```python
from build123d import *

# Parameters (mm, degrees)
F1_DEPTH = 30
F2_T     = -1
F3_DEPTH = 1


with BuildPart() as f1:
    # F0 (on Top) → F1 (new body)
    with BuildSketch(Plane.XY):
        Polygon((0, -120), (0, 0), (-25, 0), (-25, -35), (-25, -60), (-25, -100), (-25, -120), align=None)
        Polygon((0, -180), (0, -120), (-25, -120), (-25, -125), (-25, -180), align=None)
        Polygon((-25, -60), (-25, -35), (-145, -35), (-145, -60), (-110, -60), (-85, -60), align=None)
        Polygon((-25, -125), (-25, -120), (-25, -100), (-85, -100), (-85, -120), (-85, -125), align=None)
        Polygon((-85, -100), (-85, -60), (-110, -60), (-110, -120), (-85, -120), align=None)
    extrude(amount=F1_DEPTH)

    # F2
    f2_openings = [f1.faces().sort_by_distance(p)[0] for p in [
        (-12.5, -180, 15),
    ]]
    offset(amount=F2_T, openings=f2_openings, kind=Kind.INTERSECTION)

    # F3 (cut): a face of the model
    f3_faces = [f1.faces().sort_by_distance(p)[0] for p in [
        (-12.5, -2.3113848663, 30),
    ]]
    extrude(f3_faces, amount=-F3_DEPTH, mode=Mode.SUBTRACT)


solid = f1.part
```
Could you check a few things on this model? Use its own coordinates, in mm. A direction names the side the tool comes from. Round coordinates to 2 decimals unless told otherwise and drop trailing zeros. Loops run counter-clockwise (first coordinate to the right, second up) from the corner with the lowest first, then second, coordinate; pieces in that order, holes last. Notation, with made-up numbers: M 67,-3.5 L 121,-3.5 A8 ccw 121,11.5 Z; hole C -4.75,-11.75 d10. An arc over 180 degrees is marked long. Put each result on its own line as item: value.
Q1. Imagine slicing it at D-D (y = -68.5). Write out the boundary of the cut face in (x, z), then the cut area to 3 significant figures.
Check result:
outline: M -110,0 L -85,0 L -85,29 L -86,29 L -86,1 L -109,1 L -109,29 L -110,29 Z; M -25,0 L 0,0 L 0,29 L -1,29 L -1,1 L -24,1 L -24,29 L -25,29 Z
area: 162 mm2
Q2. On a 3-axis mill with a long thin cutter (end or side, diameter ignored), from which of +Z, -Z, +X, -X, +Y, -Y can I reach the whole of each face in a straight line? I mean faces 1 (the face through (-128, -60, 14)), 2 (the face through (-83, -36, 15)), 3 (the face through (-84, -35, 14)), 4 (the face through (-25, -80, 14)). Say none if no direction works.
Check result:
face 1: +Z, -Z, -X, -Y
face 2: +Z
face 3: +Z, -Z, -X, +Y
face 4: +Z, -Z
Q3. Imagine slicing it at A-A (z = 4.5). State how many separate pieces and enclosed holes the cut face has, then the cut area to 3 significant figures.
Check result:
separate pieces: 2
enclosed holes: 1
area: 827 mm2
Q4. For pin 1 (5 mm diameter, centred on y = -155.5, z = 9.5, fed in from -X); pin 2 (7.5 mm diameter, centred on x = -95.5, z = 7.5, fed in from -Y); pin 3 (14.5 mm diameter, centred on y = -74.5, z = 12, fed in from -X), each with a flat end and sliding along its axis, tell me the tip position at first contact or that it passes through.
Check result:
pin 1: x = -25
pin 2: y = -120
pin 3: x = -110
Q5. Imagine slicing it at B-B (x = -64.5). Write out the boundary of the cut face in (y, z), then the cut area to 3 significant figures.
Check result:
outline: M -125,0 L -100,0 L -100,29 L -101,29 L -101,1 L -124,1 L -124,29 L -125,29 Z; M -60,0 L -35,0 L -35,29 L -36,29 L -36,1 L -59,1 L -59,29 L -60,29 Z
area: 162 mm2
Q6. I need wall thicknesses on probe 1 along Y at (x, z) = (-38, 28); probe 2 along X at (y, z) = (-97, 8.75); probe 3 along Y at (x, z) = (-139, 26). Which ranges of each line are inside material? Lowest first, please.
Check result:
probe 1: -125 to -124, -101 to -100, -60 to -59, -36 to -35
probe 2: -110 to -109, -86 to -85, -25 to -24, -1 to 0
probe 3: -60 to -59, -36 to -35
Q7. Thinking about a two-plate mould opening in X: for faces 5 (the face through (-55, -125, 14)), 6 (the face through (-24, -80, 15)), 7 (the face through (-145, -47, 14)), which applies, released by +X, released by -X, zero draft, split by the parting line, or undercut?
Check result:
face 5: zero draft
face 6: undercut
face 7: released by -X
Q8. Imagine slicing it at C-C (y = -45.5). Write out the boundary of the cut face in (x, z).
Check result:
outline: M -145,0 L 0,0 L 0,29 L -1,29 L -1,1 L -144,1 L -144,29 L -145,29 Z
